Could you check a few things on this model? Use its own coordinates, in mm. Face numbers are marked on the shaded views. A direction names the side the tool comes from. Round coordinates to 2 decimals unless told otherwise and drop trailing zeros. Loops run counter-clockwise (first coordinate to the right, second up) from the corner with the lowest first, then second, coordinate; pieces in that order, holes last. Notation, with made-up numbers: M 85.25,66 L 93.25,66 A24 cw 93.25,96 Z; hole C 53,-6.75 d3. An arc over 180 degrees is marked long. One line per item, written item: value. Start each with the question number.
Q1. Imagine slicing it at A-A (x = 0). Please give me the cut outline in (y, z).
Q2. Which directions (+Z, -Z, +X, -X, +Y, -Y) give clear straight access to the entire face, cutting with the end or side of a thin tool? Please do the marked faces 4, 5, 6 and 7.
Q3. Thinking about a two-plate mould opening in Z: for the marked faces 1, 2 and 3, which applies, released by +Z, released by -Z, zero draft, split by the parting line, or undercut?
Q4. Imagine slicing it at D-D (y = 37.5). Please give me the cut outline in (x, z), then the cut area to 3 significant figures.
Q5. I'm going to push flat-ended pins straight in: pin 1 Ø4 at (x, z) = (13.5, 8) entering from +Y; pin 2 Ø6 at (y, z) = (45.5, 13) entering from +X; pin 3 Ø10 at (x, z) = (-4.5, 32.5) entering from -Y. Where does each tip first touch, or does it pass through?
Q6. Imagine slicing it at B-B (y = 0). Please give me the cut outline in (x, z), then the cut area to 3 significant figures.
Q7. Please list where these lines run through material, in increasing order: line 1 along Y through (x, z) = (0, 10); line 2 along X through (y, z) = (0, 7.25); line 3 along Z through (x, y) = (0, 29).
Q8. Imagine slicing it at C-C (z = 30). Please give me the cut outline in (x, y).
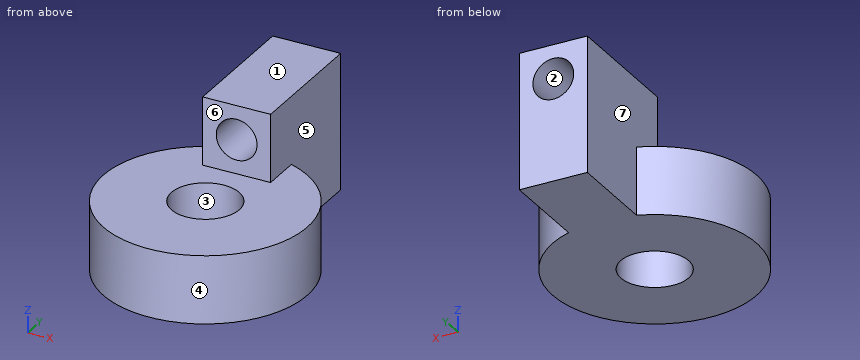
Autodesk Inventor part; units mm, degrees
ref_plane "YZ Plane" through (0, 0, 0) normal (1, 0, 0) x (0, 1, 0)
ref_plane "XZ Plane" through (0, 0, 0) normal (0, 1, 0) x (-1, 0, 0)
ref_plane "XY Plane" through (0, 0, 0) normal (0, 0, 1) x (1, 0, 0)
sketch "Sketch1" plane through (0, 0, 0) normal (0, 0, 1) x (1, 0, 0)
  circle A0 centre (0, 0) radius 30
  circle A1 centre (0, 0) radius 10
  line L0 (-30, 0) -> (30, 0)
  line L1 (30, 0) -> (30, 20)
  line L2 (30, 20) -> (-30, 20)
  line L3 (-30, 20) -> (-30, 0)
  line L4 (-10, 20) -> (10, 20)
  line L5 (10, 20) -> (10, 55)
  line L6 (10, 55) -> (-10, 55)
  line L7 (-10, 55) -> (-10, 20)
  point P0 (10, 28.2843)
  point P1 (-10, 28.2843)
  dimension "d0" = 60
  dimension "d1" = 20
  dimension "d2" = 20
  dimension "d3" = 20
  dimension "d4" = 35
extrude "Extrusion1" add sketch "Sketch1" along normal blind 40 contours L0 A1 A0 | A0 L2 L0 A1 | A0 L7 L2 | L2 L5 A0 | L7 L6 L5 A0 | A0 L5 L2 L7
sketch "Sketch2" plane through (0, 0, 40) normal (0, 0, 1) x (1, 0, 0)
  circle A0 centre (0, 0) radius 30
  line L0 (10, 55) -> (-10, 55)
  line L1 (-10, 55) -> (10, 55)
  line L2 (10, 55) -> (10, 17)
  line L3 (10, 17) -> (-10, 17)
  line L4 (-10, 17) -> (-10, 55)
  circle A1 centre (0, 0) radius 10
  point P0 (-10, 28.2843)
  point P1 (10, 28.2843)
  dimension "d7" = 38
extrude "Extrusion2" cut sketch "Sketch2" against normal blind 20 contours A0 L4 L3 L2 picked at (15.0969, 11.943)
sketch "Sketch3" plane through (-10, 55, 0) normal (0, 1, 0) x (1, 0, 0)
  circle A0 centre (10, -30) radius 6
  point P0 (10, 0)
  dimension "d10" = 12
extrude "Extrusion3" cut sketch "Sketch3" against normal blind 40.325
properties part number "End motor link"
Report:
1. outline: M -30,0 L -10,0 L -10,20 L -30,20 Z; M 10,0 L 55,0 L 55,24 L 17,24 L 17,20 L 10,20 Z; M 17,36 L 55,36 L 55,40 L 17,40 Z
2. face 4: +Z, -Z
2. face 5: +Z, +X, +Y
2. face 6: +Z, +X, -X, -Y
2. face 7: +Z, -X, +Y
3. face 1: released by +Z
3. face 2: undercut
3. face 3: zero draft
4. outline: M -10,0 L 10,0 L 10,40 L -10,40 Z; hole C 0,30 d12
4. area: 687 mm²
5. pin 1: stops at y = 27.71
5. pin 2: stops at x = 10
5. pin 3: stops at y = 17
6. outline: M -30,0 L -10,0 L -10,20 L -30,20 Z; M 10,0 L 30,0 L 30,20 L 10,20 Z
6. area: 800 mm²
7. line 1: y = -30 to -10, 10 to 55
7. line 2: x = -30 to -10, 10 to 30
7. line 3: z = 0 to 24, 36 to 40
8. outline: M -10,17 L -6,17 L -6,55 L -10,55 Z; M 6,17 L 10,17 L 10,55 L 6,55 Z
